The listing builds one solid part. Answer for the finished solid, in the listing's coordinates (mm). A direction names the side the tool comes from. Round coordinates to 2 decimals unless told otherwise and drop trailing zeros. Write each loop counter-clockwise with the first axis right and the second up, starting at its lowest first coordinate (ties: lowest second). Pieces come first, ordered by that corner, then holes.
Item 1: Find section C-C on z = 0. Give the number of separate pieces and of enclosed holes in the cut face, then the cut area to 3 significant figures.
Item 2: Each of these flat-tipped pins is pushed along its axis until it touches: pin 1 (16 mm diameter, centred on y = 23.454, z = 30, fed in from -X); pin 2 (10 mm diameter, centred on x = 46, y = -5.5, fed in from +Z); pin 3 (11 mm diameter, centred on x = 38.88, z = 0, fed in from -Y); pin 4 (2 mm diameter, centred on y = 13.5, z = 0.5, fed in from -X). Where does it stop, or does it pass through?
Item 3: Find section B-B on y = 55. Give the vertices of the cut face in (x, z), then the cut area to 3 significant figures.
Item 4: Find section A-A on z = 28. Give the vertices of the cut face in (x, y).
Item 5: Find section D-D on y = -20. Give the vertices of the cut face in (x, z).
Item 6: A tool of negligible diameter and unlimited length cuts with its end or side. For faces 4 (the face through (35.68, -39.18, -16.27)), 5 (the face through (80.28, -27.99, 3.9)), 6 (the face through (35.8, -39.18, 16.38)), 7 (the face through (8.77, 42.53, 6.01)), from which of +Z, -Z, +X, -X, +Y, -Y can it reach the whole face along a straight path? Write none if from no direction.
Item 7: Find the intervals of material crossed by probe 1 along X at (y, z) = (-3.5, 9); probe 2 along X at (y, z) = (44.5, 30); probe 3 along Y at (x, z) = (-23.25, -30), in increasing order.
Item 8: For a pull along X with two mould halves and no side action, classify faces 1 (the face through (23.88, -39.18, -0.21)), 2 (the face through (67, -33.755, 24)), 3 (the face through (-16.987, 42.68, -6.054)) as +X half, -X half, draft (parallel to the pull), parting line (faces both ways), or undercut.
Autodesk Inventor part; units mm, degrees
ref_plane "Work Plane1" through (-19.05, 0, 0) normal (1, 0, 0) x (0, 1, 0)
ref_plane "XZ Plane" through (0, 0, 0) normal (0, 1, 0) x (-1, 0, 0)
ref_plane "XY Plane" through (0, 0, 0) normal (0, 0, 1) x (1, 0, 0)
sketch "Sketch1" plane through (0, 0, 0) normal (0, 0, 1) x (1, 0, 0)
  line L0 (-244.3747, 73.9364) -> (-91.8552, 73.9364) construction
  line L1 (-91.8552, 73.9364) -> (-91.8552, -48.2612) construction
  line L2 (-91.8552, -48.2612) -> (-244.3747, -48.2612) construction
  line L3 (-244.3747, -48.2612) -> (-244.3747, 73.9364) construction
  line L4 (-19.331, 24.2448) -> (33.669, 24.2448)
  line L5 (68.669, -10.7552) -> (68.669, -33.7552)
  arc A0 (68.669, -10.7552) -> (33.669, 24.2448) centre (33.669, -10.7552) ccw
  point P0 (0, 0)
  dimension "d13" = 58
  dimension "d15" = 35
ref_plane "Work Plane1" through (-19.05, 0, 0) normal (1, 0, 0) x (0, 1, 0)
sketch "Sketch2" plane through (-19.05, 0, 0) normal (1, 0, 0) x (0, 1, 0)
  point P0 (0, 0)
sketch "Sketch3" plane through (-19.05, 0, 0) normal (1, 0, 0) x (0, 1, 0)
  circle A0 centre (23.454, 0) radius 20
  point P0 (0, 0)
  dimension "d16" = 40
sweep "Sweep1" add profiles "Sketch3" path "Sketch1"
shell "Shell1" thickness 7 removed faces 2 at (-19.331, 19.2276, 1.3227) at (61.9752, -33.7552, -3.0982)
sketch "Sketch4" plane through (-19.331, 23.454, 0) normal (-1, 0, 0) x (0, 0, 1)
  point P0 (0, -23.454)
sketch "Sketch5" plane through (-19.331, 23.454, 0) normal (-1, 0, 0) x (0, 0, 1)
  point P0 (0, -23.454)
sketch "Sketch6" plane through (-19.331, 23.454, 0) normal (-1, 0, 0) x (0, 0, 1)
  point P0 (0, -23.454)
sketch "Sketch7" plane through (-19.331, 23.454, 0) normal (-1, 0, 0) x (0, 0, 1)
  point P0 (0, -23.454)
sketch "Sketch8" plane through (-19.331, 23.454, 0) normal (-1, 0, 0) x (0, 0, 1)
  point P0 (0, -23.454)
sketch "Sketch9" plane through (-19.331, 23.454, 0) normal (-1, 0, 0) x (0, 0, 1)
  point P0 (0, -23.454)
sketch "Sketch10" plane through (-19.331, 23.454, 0) normal (-1, 0, 0) x (0, 0, 1)
  point P0 (0, -23.454)
sketch "Sketch11" plane through (-19.331, 23.454, 0) normal (-1, 0, 0) x (0, 0, 1)
  point P0 (0, -23.454)
sketch "Sketch12" plane through (-19.331, 23.454, 0) normal (-1, 0, 0) x (0, 0, 1)
  point P0 (0, -23.454)
sketch "Sketch13" plane through (-19.331, 23.454, 0) normal (-1, 0, 0) x (0, 0, 1)
  point P0 (0, -23.454)
sketch "Sketch14" plane through (-19.331, 23.454, 0) normal (-1, 0, 0) x (0, 0, 1)
  point P0 (0, -23.454)
sketch "Sketch15" plane through (-19.331, 23.454, 0) normal (-1, 0, 0) x (0, 0, 1)
  point P0 (0, -23.454)
sketch "Sketch16" plane through (-19.331, 23.454, 0) normal (-1, 0, 0) x (0, 0, 1)
  circle A0 centre (0, 0) radius 39
  circle A1 centre (0, 0) radius 13
  point P0 (0, -23.454)
  dimension "d20" = 78
  dimension "d21" = 26
extrude "Extrusion1" add sketch "Sketch16" along normal blind 8
sketch "Sketch17" plane through (-27.331, 23.454, 0) normal (-1, 0, 0) x (0, 0, 1)
  circle A0 centre (0, 30) radius 5
  circle A1 centre (0, 0) radius 13
  circle A2 centre (-30, 0) radius 5
  circle A3 centre (0, -30) radius 5
  circle A4 centre (30, 0) radius 5
  point P0 (0, -23.454)
  dimension "d24" = 10
  dimension "d25" = 30
  dimension "d28" = 360
extrude "Extrusion2" cut sketch "Sketch17" against normal blind 8 contours A0 | A2 | A3 | A4
chamfer "Chamfer1" distance 2.5 angle 45 1 edges at (-19.331, 3.454, 0)
sketch "Sketch18" plane through (67.8782, -33.7552, 0) normal (0, -1, 0) x (1, 0, 0)
  circle A0 centre (0, 0) radius 13
  circle A1 centre (0, 0) radius 13
  circle A2 centre (29, 0) radius 6
  arc A3 (36.8103, -12.8062) -> (36.8103, 12.8062) centre (29, 0) ccw
  arc A4 (28.2321, 20.6869) -> (36.8103, 12.8062) centre (52.431, 38.4186) ccw
  arc A5 (36.8103, -12.8062) -> (28.2321, -20.6869) centre (52.431, -38.4186) ccw
  circle A6 centre (-29, 0) radius 6
  arc A7 (-36.8103, 12.8062) -> (-36.8103, -12.8062) centre (-29, 0) ccw
  arc A8 (-36.8103, 12.8062) -> (-28.2321, 20.6869) centre (-52.431, 38.4186) ccw
  arc A9 (-28.2321, -20.6869) -> (-36.8103, -12.8062) centre (-52.431, -38.4186) ccw
  arc A10 (28.2321, 20.6869) -> (-28.2321, 20.6869) centre (0, 0) ccw
  arc A11 (-28.2321, -20.6869) -> (28.2321, -20.6869) centre (0, 0) ccw
  point P0 (-67.8782, 0)
  dimension "d36" = 26
  dimension "d38" = 12
  dimension "d39" = 29
  dimension "d41" = 30
  dimension "d42" = 29
extrude "Extrusion3" add sketch "Sketch18" along normal blind 11
chamfer "Chamfer2" distance 2.5 angle 45 1 edges at (47.8782, -33.7552, 0)
properties part number "cad@41"
Check values:
1. separate pieces: 6
1. enclosed holes: 0
1. area: 2,500 mm2
2. pin 1: stops at x = -27.33
2. pin 2: stops at z = 12.26
2. pin 3: stops at y = -1.42
2. pin 4: stops at x = 73.54
3. outline: (-27.33, -22.93) - (-19.33, -22.93) - (-19.33, -4.75) - (-27.33, -4.75) - close; (-27.33, 4.75) - (-19.33, 4.75) - (-19.33, 22.93) - (-27.33, 22.93) - close
3. area: 291 mm2
4. outline: (-27.33, -3.69) - (-19.33, -3.69) - (-19.33, 18.87) - (-27.33, 18.87) - close; (-27.33, 28.04) - (-19.33, 28.04) - (-19.33, 50.6) - (-27.33, 50.6) - close; (46.88, -44.76) - (88.88, -44.76) - (88.88, -33.76) - (46.88, -33.76) - close
5. outline: circle Ø40 at (67.88, 0); hole circle Ø26 at (67.88, 0)
6. face 4: -Z, -X, -Y
6. face 5: -Y
6. face 6: +Z, -X, -Y
6. face 7: none
7. probe 1: x = -27.33 to -19.33, 48.32 to 57.41, 76.65 to 85.23
7. probe 2: x = -27.33 to -19.33
7. probe 3: y = -1.47 to 18.45, 28.45 to 48.37
8. face 1: -X half
8. face 2: draft
8. face 3: undercut
